```python
from build123d import *

# Parameters (mm, degrees)
F0_W     = 400
F0_H     = 200
F1_DEPTH = 150
F2_W     = 360
F2_H     = 160
F3_DEPTH = 130
F4_R     = 5
F5_DEPTH = 20


with BuildPart() as f1:
    # F0 (on Top) → F1 (new body)
    with BuildSketch(Plane.XY):
        Rectangle(F0_W, F0_H)
    extrude(amount=F1_DEPTH)

    # F2 (on face) → F3 (cut)
    with BuildSketch(Plane.XY.offset(150)):
        Rectangle(F2_W, F2_H)
    extrude(amount=-F3_DEPTH, mode=Mode.SUBTRACT)

    # F4 (on face) → F5 (cut)
    with BuildSketch(Plane.XY.offset(150)):
        with Locations((-150, 90)):
            Circle(F4_R)
        with Locations((-110, 90)):
            Circle(F4_R)
        with Locations((110, 90)):
            Circle(F4_R)
        with Locations((150, 90)):
            Circle(F4_R)
    extrude(amount=-F5_DEPTH, mode=Mode.SUBTRACT)


solid = f1.part
```
Source: CAD feature listing. Evaluate the final solid. Frame: model axes, mm. A direction names the side the tool comes from. Give positions to 0.01 mm unless a question says otherwise; leave off trailing zeros. Loops run counter-clockwise (first coordinate to the right, second up) from the corner with the lowest first, then second, coordinate; pieces in that order, holes last. Notation, with made-up numbers: (-35.5, -8) - (-6.5, -8) arc R15 ccw to (-6.5, 9) - close; hole circle Ø1 at (68.25, 6). An arc over 180 degrees is marked (long way). Use CSV: the item, a comma, the result in double quotes.
1) Cut plane D-D (x = 110). Output: boundary loops of the cut face in (y, z).
Worked out:
outline,"(-100, 0) - (100, 0) - (100, 150) - (95, 150) - (95, 130) - (85, 130) - (85, 150) - (80, 150) - (80, 20) - (-80, 20) - (-80, 150) - (-100, 150) - close"
2) Set-up query: faces 4 (the flat face through (-16, -81, 150)), 5 (the cylindrical face through (-154, 87, 140)). Return all of +Z, -Z, +X, -X, +Y, -Y with unobstructed straight access to the full face (end or side cutting, diameter ignored); none if empty.
Worked out:
face 4,"+Z, +X, -X, +Y, -Y"
face 5,"+Z"
3) Line query: line 1 (Y direction, x = 150, z = 146); line 2 (X direction, y = 40, z = 112); line 3 (Y direction, x = 0, z = 107). Output: solid intervals per line, ascending.
Worked out:
line 1,"y = -100 to -80, 80 to 85, 95 to 100"
line 2,"x = -200 to -180, 180 to 200"
line 3,"y = -100 to -80, 80 to 100"
4) Cut plane A-A (z = 29.5). Output: boundary loops of the cut face in (x, y), and give its area (3 significant figures).
Worked out:
outline,"(-200, -100) - (200, -100) - (200, 100) - (-200, 100) - close; hole (-180, -80) - (180, -80) - (180, 80) - (-180, 80) - close"
area,"22,400 mm^2"
5) Cut plane C-C (x = 5.5). Output: boundary loops of the cut face in (y, z), and give its area (3 significant figures).
Worked out:
outline,"(-100, 0) - (100, 0) - (100, 150) - (80, 150) - (80, 20) - (-80, 20) - (-80, 150) - (-100, 150) - close"
area,"9,200 mm^2"
6) Pin query (flat end, axial travel): P1, Ø6, axis at x = -150, y = 90, coming from the -Z side; P2, Ø6, axis at x = -110, y = 90, coming from the +Z side; P3, Ø8, axis at x = -112, y = -9, coming from the +Z side. Return the tip coordinate at first contact, or that it passes through.
Worked out:
P1,"stops at z = 0"
P2,"stops at z = 130"
P3,"stops at z = 20"
7) Mould query, pull axis X, two halves, no side actions, for faces 1 (the flat face through (-3, -100, 74)), 2 (the flat face through (-3, 1, 20)), 3 (the flat face through (200, -1, 74)). Classes: +X half, -X half, draft (parallel to the pull), parting line (faces both ways), or undercut.
Worked out:
face 1,"draft"
face 2,"undercut"
face 3,"+X half"
8) Cut plane B-B (y = 35). Output: boundary loops of the cut face in (x, z), and give its area (3 significant figures).
Worked out:
outline,"(-200, 0) - (200, 0) - (200, 150) - (180, 150) - (180, 20) - (-180, 20) - (-180, 150) - (-200, 150) - close"
area,"13,200 mm^2"
